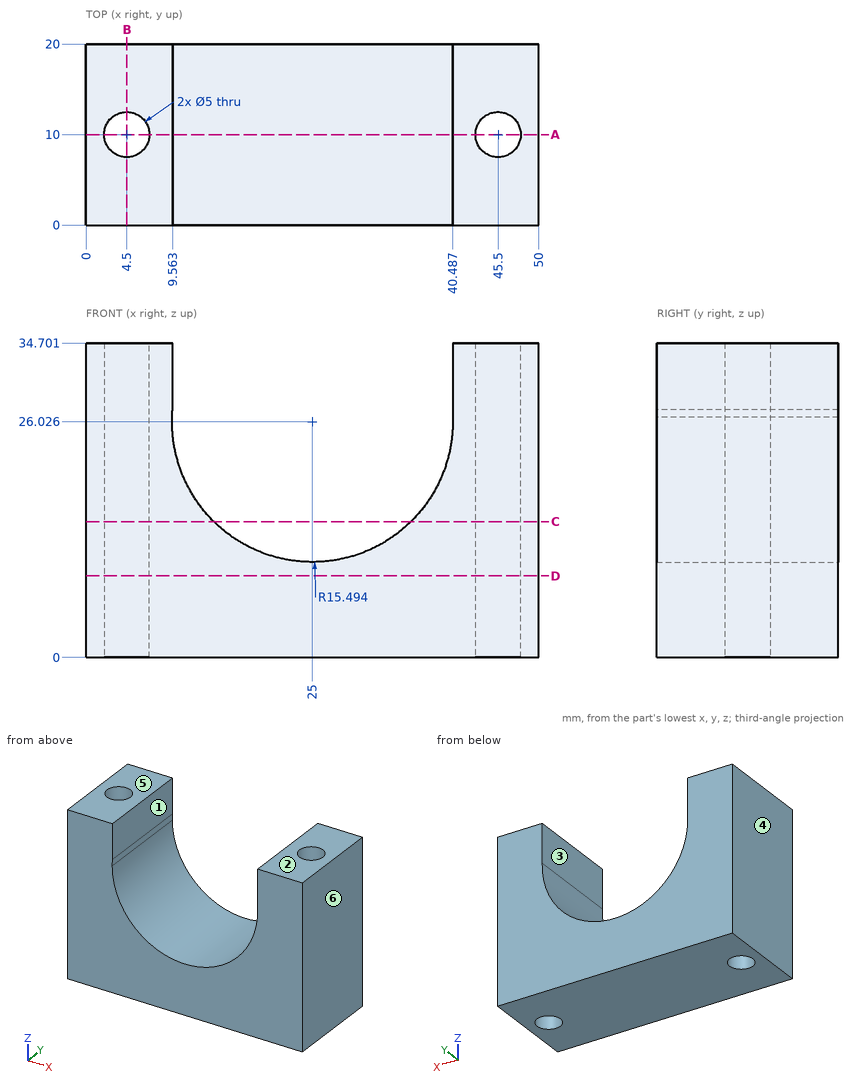
Geometry: see drawing. Coordinates: mm, zero at the bounding-box minimum. A direction names the side the tool comes from. Round coordinates to 2 decimals unless told otherwise and drop trailing zeros. Loops run counter-clockwise (first coordinate to the right, second up) from the corner with the lowest first, then second, coordinate; pieces in that order, holes last. Notation, with made-up numbers: (-25, -14) - (32, -14) arc R26 cw to (32, 17) - close; hole circle Ø9 at (79, 41.5). An arc over 180 degrees is marked (long way). Write item = value, one per line. Start each with the question number.
(1) Ray query, line 1 along Y through (x, z) = (4.5, 13); line 2 along X through (y, z) = (10, 24.5); line 3 along X through (y, z) = (11.5, 14.5) (1 decimal). Return the intervals inside material, ascending. Write a range as from..to.
(2) Pin query (flat end, axial travel): pin 1 (1.5 mm diameter, centred on x = 29, z = 13, fed in from -Y). Return the tip coordinate at first contact, or that it passes through.
(3) Section query B-B, the plane x = 4.5. Output: boundary loops of the cut face in (y, z).
(4) Set-up query: the marked faces 1 and 2. Return all of +Z, -Z, +X, -X, +Y, -Y with unobstructed straight access to the full face (end or side cutting, diameter ignored); none if empty.
(5) Section query D-D, the plane z = 9. Output: boundary loops of the cut face in (x, y).
(6) Section query A-A, the plane y = 10. Output: boundary loops of the cut face in (x, z) (1 decimal).
(7) Pull-direction query (X, two-part tool) for the marked faces 3, 4, 5 and 6; classes: +X half, -X half, draft (parallel to the pull), parting line (faces both ways), or undercut.
(8) Section query C-C, the plane z = 15. Output: boundary loops of the cut face in (x, y).
Conclusion:
q1.line_1 = 0..7.5, 12.5..20
q1.line_2 = 0..2, 7..9.58, 40.42..43, 48..50
q1.line_3 = 0..2.5, 6.5..14.6, 35.4..43.5, 47.5..50
q2.pin_1 = through
q3.outline = (0, 0) - (7.5, 0) - (7.5, 34.7) - (0, 34.7) - close; (12.5, 0) - (20, 0) - (20, 34.7) - (12.5, 34.7) - close
q4.face_1 = +Z, +Y, -Y
q4.face_2 = +Z, +X, -X, +Y, -Y
q5.outline = (0, 0) - (50, 0) - (50, 20) - (0, 20) - close; hole circle Ø5 at (4.5, 10); hole circle Ø5 at (45.5, 10)
q6.outline = (0, 0) - (2, 0) - (2, 34.7) - (0, 34.7) - close; (7, 0) - (43, 0) - (43, 34.7) - (40.5, 34.7) - (40.5, 26.5) arc R15.5 cw (long way) to (9.6, 27.4) - (9.6, 34.7) - (7, 34.7) - close; (48, 0) - (50, 0) - (50, 34.7) - (48, 34.7) - close
q7.face_3 = undercut
q7.face_4 = -X half
q7.face_5 = draft
q7.face_6 = +X half
q8.outline = (0, 0) - (14.11, 0) - (14.11, 20) - (0, 20) - close; (35.89, 0) - (50, 0) - (50, 20) - (35.89, 20) - close; hole circle Ø5 at (4.5, 10); hole circle Ø5 at (45.5, 10)
